Drawing for the job (mm, zero at the part's lowest x, y, z). A direction names the side the tool comes from. Coordinates: 2 decimals unless noted, no trailing zeros. Loops run counter-clockwise (first coordinate to the right, second up) from the corner with the lowest first, then second, coordinate; pieces in that order, holes last. Notation, with made-up numbers: (8, 35) -> (29, 35) arc R12 cw to (29, 49) -> close; hole circle Ø5 at (53, 53.25). An arc over 180 degrees is marked (long way). Write item = value, one per line. Start each with the question number.
(1) Tool access for the marked faces 4, 5 and 6: list every direction of +Z, -Z, +X, -X, +Y, -Y with a clear straight run to the whole face (end or side of a thin tool).
(2) Band-saw the part on D-D (z = 15). Write the cut outline in (x, y).
(3) Flat gauge pins, fed straight in: P1, Ø3, axis at x = 7.5, y = 6, coming from the +Z side; P2, Ø4, axis at x = 10, z = 24.39, coming from the +Y side; P3, Ø12, axis at x = 13.5, z = 14.5, coming from the -Y side; P4, Ø0.5, axis at y = 0.5, z = 22, coming from the +X side. Where does each tip first touch, or does it go through?
(4) Drill centre lines: line 1 (Z direction, x = 10, y = 0.3); line 2 (Z direction, x = 17.5, y = 1.75); line 3 (Y direction, x = 14, z = 11.5). Where is each one in solid material? Low to high. Write a range as from..to.
(5) Band-saw the part on C-C (x = 4). Write the cut outline in (y, z).
(6) Band-saw the part on A-A (y = 4.75). Write the cut outline in (x, z).
(7) Pull direction Z, two halves, no side cores. Call the marked faces 1, 2 and 3: +Z half, -Z half, draft (parallel to the pull), parting line (faces both ways), or undercut.
(8) Band-saw the part on B-B (x = 10). Write the cut outline in (y, z).
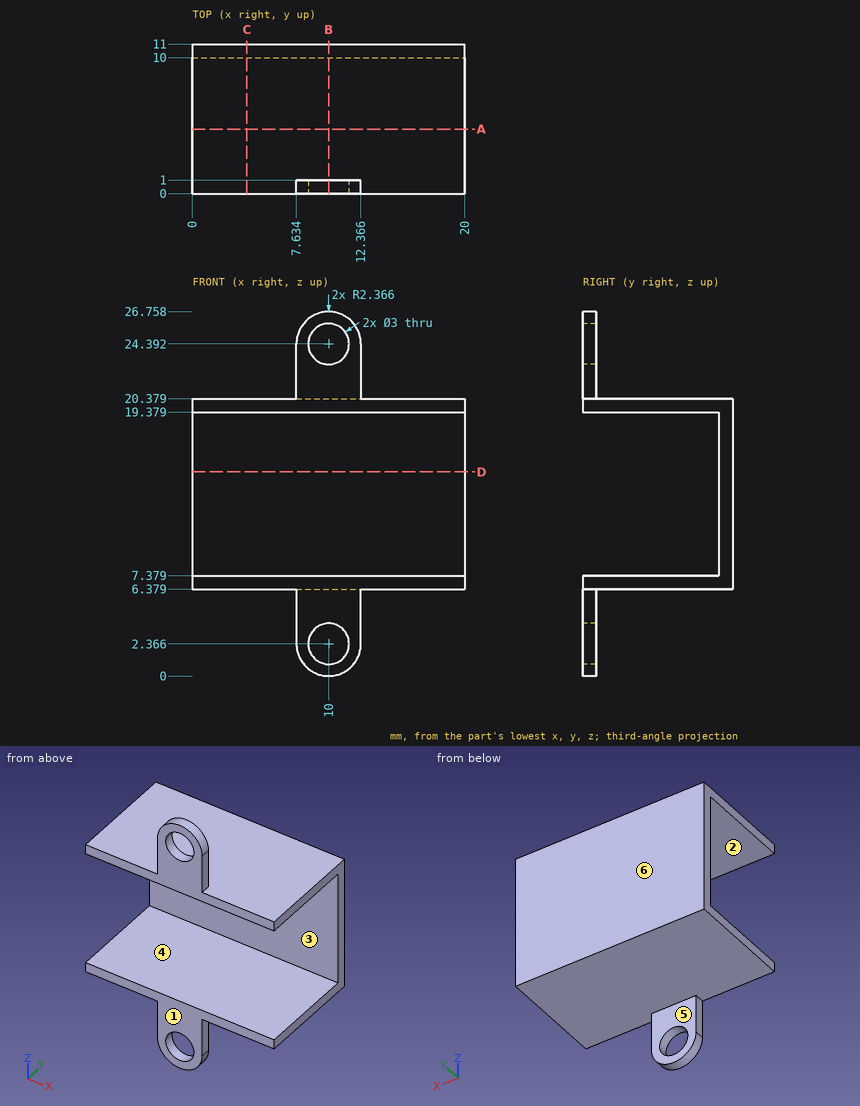
Findings below:
q1.face_4 = +X, -X, -Y
q1.face_5 = -Z, +X, -X, +Y
q1.face_6 = +Z, -Z, +X, -X, +Y
q2.outline = (0, 10) -> (20, 10) -> (20, 11) -> (0, 11) -> close
q3.P1 = 20.38
q3.P2 = 1
q3.P3 = 0
q3.P4 = 12.37
q4.line_1 = 0..0.87, 3.87..7.38, 19.38..22.89, 25.89..26.76
q4.line_2 = 6.38..7.38, 19.38..20.38
q4.line_3 = 10..11
q5.outline = (0, 6.38) -> (11, 6.38) -> (11, 20.38) -> (0, 20.38) -> (0, 19.38) -> (10, 19.38) -> (10, 7.38) -> (0, 7.38) -> close
q6.outline = (0, 6.38) -> (20, 6.38) -> (20, 7.38) -> (0, 7.38) -> close; (0, 19.38) -> (20, 19.38) -> (20, 20.38) -> (0, 20.38) -> close
q7.face_1 = draft
q7.face_2 = undercut
q7.face_3 = undercut
q8.outline = (0, 0) -> (1, 0) -> (1, 0.87) -> (0, 0.87) -> close; (0, 3.87) -> (1, 3.87) -> (1, 6.38) -> (11, 6.38) -> (11, 20.38) -> (1, 20.38) -> (1, 22.89) -> (0, 22.89) -> (0, 19.38) -> (10, 19.38) -> (10, 7.38) -> (0, 7.38) -> close; (0, 25.89) -> (1, 25.89) -> (1, 26.76) -> (0, 26.76) -> close
